Could you check a few things on this drawing? It's one solid part, dimensions in mm from its lowest x, y, z. A direction names the side the tool comes from. Give positions to 0.01 mm unless a question says otherwise; leave off trailing zeros. Order: outer loops, then holes, each group sorted by start corner. A loop starts at its lowest first (then second) coordinate and runs counter-clockwise, first axis right, second up.
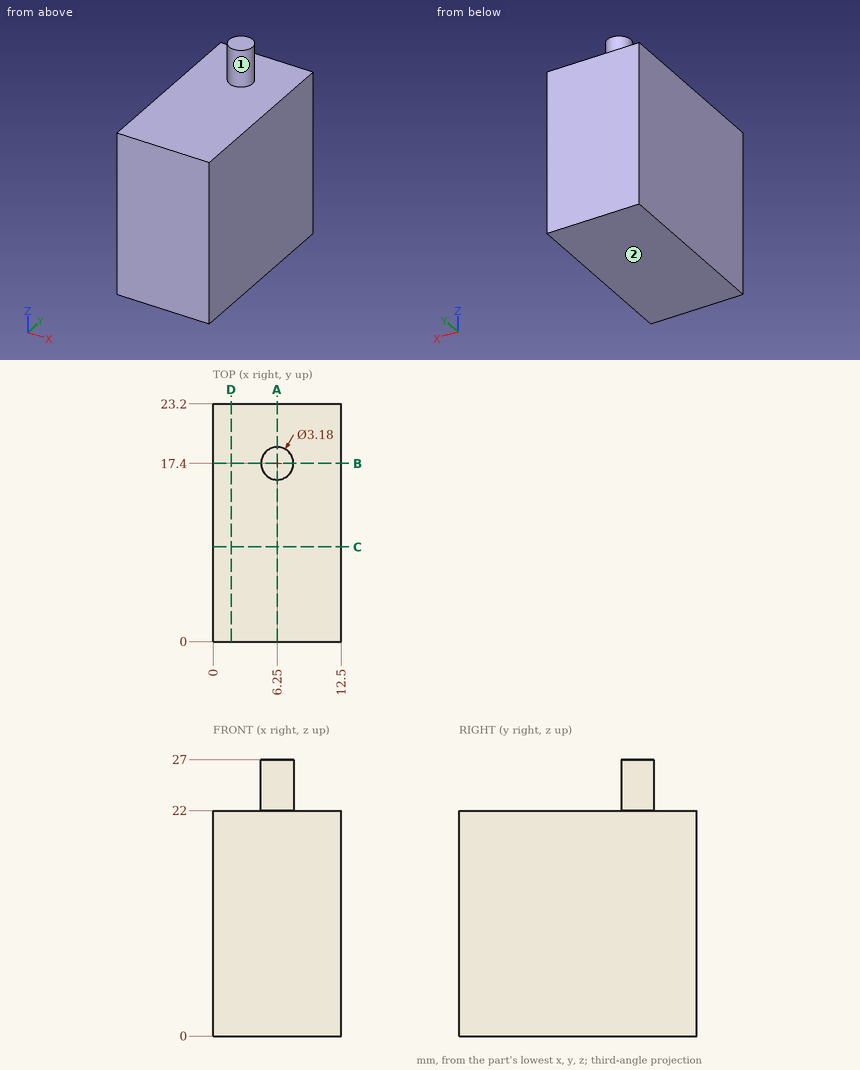
Item 1: For the marked faces 1 and 2, which set-ups out of +Z, -Z, +X, -X, +Y, -Y let a thin tool reach every point of the face, with its end or its side?
Findings:
face 1: +Z
face 2: -Z, +X, -X, +Y, -Y
Item 2: Please list where this line runs through material, in increasing order: line 1 along Z through (x, y) = (11, 21).
Findings:
line 1: z = 0 to 22
Item 3: Imagine slicing it at A-A on x = 6.25. List the corners of the cut face in (y, z) for me, then the cut area to 3 significant figures.
Findings:
outline: (0, 0) - (23.2, 0) - (23.2, 22) - (18.99, 22) - (18.99, 27) - (15.81, 27) - (15.81, 22) - (0, 22) - close
area: 526 mm2
Item 4: Imagine slicing it at B-B on y = 17.4. List the corners of the cut face in (x, z) for me, then the cut area to 3 significant figures.
Findings:
outline: (0, 0) - (12.5, 0) - (12.5, 22) - (7.84, 22) - (7.84, 27) - (4.66, 27) - (4.66, 22) - (0, 22) - close
area: 291 mm2
Item 5: For pin 1 (4 mm diameter, centred on x = 9, y = 14.5, fed in from +Z), with a flat end and sliding along its axis, tell me the tip position at first contact or that it passes through.
Findings:
pin 1: stops at z = 22
Item 6: Imagine slicing it at C-C on y = 9.25. List the corners of the cut face in (x, z) for me.
Findings:
outline: (0, 0) - (12.5, 0) - (12.5, 22) - (0, 22) - close
Item 7: Imagine slicing it at D-D on x = 1.75. List the corners of the cut face in (y, z) for me, then the cut area to 3 significant figures.
Findings:
outline: (0, 0) - (23.2, 0) - (23.2, 22) - (0, 22) - close
area: 510 mm2
